Study the drawing (mm; zero at the part's minimum x, y, z) and answer. A direction names the side the tool comes from. Give positions to 0.01 mm unless a question says otherwise; leave off trailing zeros. Order: outer loops, then holes, each group sorted by start corner. A loop starts at its lowest first (then second) coordinate and runs counter-clockwise, first axis right, second up. Notation, with made-up numbers: (7.25, 54.5) - (46.25, 54.5) arc R18 cw to (46.25, 83.5) - close; hole circle Ø3 at (1, 51.5). An arc over 180 degrees is marked (long way). Return JSON: item names as keys, results as strings.
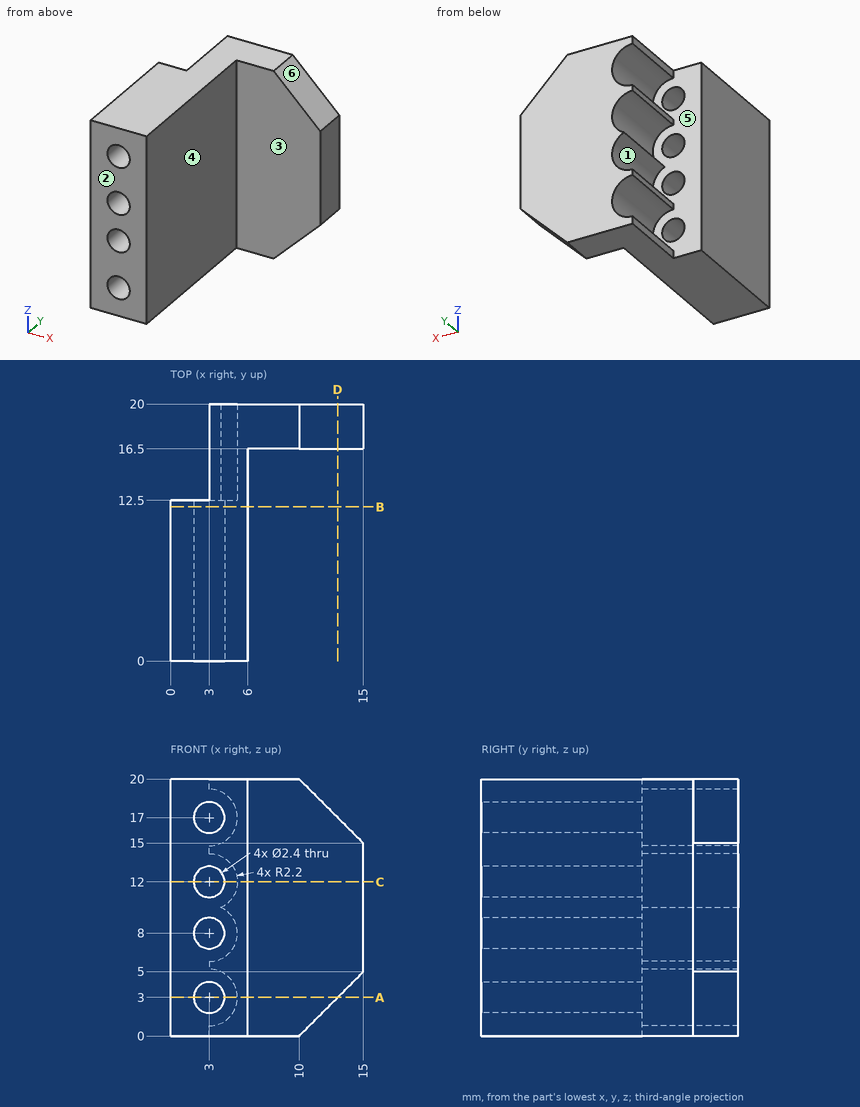
Q1. A cutting plane is placed at A-A (z = 3). Write down the section's boundary in (x, y).
Values:
{"outline": "(0, 0) - (1.8, 0) - (1.8, 12.5) - (0, 12.5) - close; (4.2, 0) - (6, 0) - (6, 16.5) - (13, 16.5) - (13, 20) - (5.2, 20) - (5.2, 12.5) - (4.2, 12.5) - close"}
Q2. Given pin 1 (0.9 mm diameter, centred on y = 15, z = 0.5, fed in from -X); pin 2 (2 mm diameter, centred on y = 17.5, z = 2.5, fed in from -X); pin 3 (8 mm diameter, centred on y = 13, z = 2, fed in from +X), each flat-ended and moving along its own axis, determine where each tip first touches the part or whether it passes through.
Values:
{"pin 1": "stops at x = 3", "pin 2": "stops at x = 4.61", "pin 3": "stops at x = 13.94"}
Q3. For the marked faces 1, 2 and 3, determine the directions among +Z, -Z, +X, -X, +Y, -Y from which every point of the face is accessible in a straight line to the end or side of a thin tool.
Values:
{"face 1": "-X, +Y", "face 2": "+Z, -Z, +X, -X, -Y", "face 3": "+Z, -Z, +X, -Y"}
Q4. Determine the mould class of the marked faces 4, 5 and 6 for opening direction Z: released by +Z, released by -Z, zero draft, split by the parting line, or undercut.
Values:
{"face 4": "zero draft", "face 5": "undercut", "face 6": "released by +Z"}
Q5. A cutting plane is placed at B-B (y = 12). Write down the section's boundary in (x, z), and give its area (3 significant figures).
Values:
{"outline": "(0, 0) - (6, 0) - (6, 20) - (0, 20) - close; hole circle Ø2.4 at (3, 3); hole circle Ø2.4 at (3, 8); hole circle Ø2.4 at (3, 12); hole circle Ø2.4 at (3, 17)", "area": "102 mm²"}
Q6. Consider L1, parallel to Z at x = 3, y = 9.25; L2, parallel to X at y = 6.25, z = 12; L3, parallel to Y at x = 4.75, z = 3.5. Determine where each line is inside the solid, lowest interval first.
Values:
{"L1": "z = 0 to 1.8, 4.2 to 6.8, 9.2 to 10.8, 13.2 to 15.8, 18.2 to 20", "L2": "x = 0 to 1.8, 4.2 to 6", "L3": "y = 0 to 12.5"}
Q7. A cutting plane is placed at C-C (z = 12). Write down the section's boundary in (x, y), and give its area (3 significant figures).
Values:
{"outline": "(0, 0) - (1.8, 0) - (1.8, 12.5) - (0, 12.5) - close; (4.2, 0) - (6, 0) - (6, 16.5) - (15, 16.5) - (15, 20) - (5.2, 20) - (5.2, 12.5) - (4.2, 12.5) - close", "area": "82.5 mm²"}
Q8. A cutting plane is placed at D-D (x = 13). Write down the section's boundary in (y, z).
Values:
{"outline": "(16.5, 3) - (20, 3) - (20, 17) - (16.5, 17) - close"}
